Build history of the part. All positions in model axes, mm. A direction names the side the tool comes from. Round coordinates to 2 decimals unless told otherwise and drop trailing zeros. Write each loop counter-clockwise with the first axis right and the second up, starting at its lowest first coordinate (ties: lowest second). Pieces come first, ordered by that corner, then holes. Notation, with made-up numbers: (-26, -34) -> (8, -34) arc R11 cw to (8, -20) -> close; hole circle Ø3 at (-12, 38.5). An arc over 180 degrees is marked (long way). Return JSON: item names as keys, results as strings.
from build123d import *

# Parameters (mm, degrees)
SKETCH1_R           = 12
BOSS_EXTRUDE1_DEPTH = 2.94
CUT_EXTRUDE1_DEPTH  = 2.94
CUT_EXTRUDE2_DEPTH  = 2.94
SKETCH7_R           = 0.5
BOSS_EXTRUDE4_DEPTH = 9.45
SKETCH8_R           = 0.6
BOSS_EXTRUDE5_DEPTH = 0.8
SKETCH9_R           = 0.35
BOSS_EXTRUDE6_DEPTH = 0.4
SKETCH10_R          = 0.085
BOSS_EXTRUDE7_DEPTH = 0.4


with BuildPart() as part:
    # Sketch1 → Boss-Extrude1 (new body)
    with BuildSketch(Plane(origin=(0, 0, 0), x_dir=(1, 0, 0), z_dir=(0, 1, 0))):
        Circle(SKETCH1_R)
    extrude(amount=BOSS_EXTRUDE1_DEPTH)

    # Sketch2 → Cut-Extrude1 (cut)
    with BuildSketch(Plane(origin=(0, 0, 0), x_dir=(1, 0, 0), z_dir=(0, 1, 0))):
        Polygon((-11.3, 0), (-11.3, 4.756450674), (-12.628390715, 4.756450674), (-12.628390715, -4.839844075), (-11.3, -4.839844075), align=None)
        Polygon((12.628390715, -4.839844075), (12.628390715, 4.756450674), (11.3, 4.756450674), (11.3, 0), (11.3, -4.839844075), align=None)
    extrude(amount=CUT_EXTRUDE1_DEPTH, mode=Mode.SUBTRACT)

    # Sketch3 → Cut-Extrude2 (cut)
    with BuildSketch(Plane(origin=(0, 0, 0), x_dir=(1, 0, 0), z_dir=(0, 1, 0))):
        Polygon((0, -11.3), (4.998184115, -11.3), (4.998184115, -12.991968643), (-5.196787457, -12.991968643), (-5.196787457, -11.3), align=None)
        Polygon((-5.196787457, 12.991968643), (4.998184115, 12.991968643), (4.998184115, 11.3), (0, 11.3), (-5.196787457, 11.3), align=None)
    extrude(amount=CUT_EXTRUDE2_DEPTH, mode=Mode.SUBTRACT)

    # Sketch7 → Boss-Extrude4 (add)
    with BuildSketch(Plane(origin=(11.3, 0, 0), x_dir=(0, 0, -1), z_dir=(1, 0, 0))):
        with Locations((0, 1.58)):
            Circle(SKETCH7_R)
    extrude(amount=BOSS_EXTRUDE4_DEPTH)

    # Sketch8 → Boss-Extrude5 (add)
    with BuildSketch(Plane(origin=(0, 2.94, 0), x_dir=(1, 0, 0), z_dir=(0, 1, 0))):
        Circle(SKETCH8_R)
    extrude(amount=BOSS_EXTRUDE5_DEPTH)

    # Sketch9 → Boss-Extrude6 (add)
    with BuildSketch(Plane(origin=(0, 3.74, 0), x_dir=(1, 0, 0), z_dir=(0, 1, 0))):
        Circle(SKETCH9_R)
    extrude(amount=BOSS_EXTRUDE6_DEPTH)

    # Sketch10 → Boss-Extrude7 (add)
    with BuildSketch(Plane(origin=(0, 4.14, 0), x_dir=(1, 0, 0), z_dir=(0, 1, 0))):
        Circle(SKETCH10_R)
    extrude(amount=BOSS_EXTRUDE7_DEPTH)


solid = part.part
Q1. Wall check: L1, parallel to X at y = 0.6, z = -0.5; L2, parallel to Y at x = 7, z = -6; L3, parallel to Z at x = 17, y = 1.5. Give the ranges that are in metal, low to high.
Verdict:
{"L1": "x = -11.3 to 11.3", "L2": "y = 0 to 2.94", "L3": "z = -0.49 to 0.49"}
Q2. Pin check, flat tips, straight feed: pin 1 Ø2 at (x, y) = (8.5, 4) entering from +Z; pin 2 Ø4 at (x, z) = (-0.5, 3) entering from +Y; pin 3 Ø11.5 at (x, z) = (5.5, -2.5) entering from +Y; pin 4 Ø2 at (x, y) = (10, 2.5) entering from -Z. Stop position of each tip, or through.
Verdict:
{"pin 1": "passes through", "pin 2": "stops at y = 2.94", "pin 3": "stops at y = 4.14", "pin 4": "stops at z = -7.94"}
Q3. Saw through at C-C on x = 18. List the corners of the cut face in (y, z).
Verdict:
{"outline": "circle Ø1 at (1.58, 0)"}
Q4. 3-axis set-ups, long thin cutter, end or side, ignore diameter. For faces 1 (the cylindrical face through (15.959, 2.076, 0.065)), 2 (the cylindrical face through (0.323, 3.334, -0.506)), 3 (the cylindrical face through (8.54, 1.45, -8.43)): which of +Z, -Z, +X, -X, +Y, -Y reach the whole face in a straight line?
Verdict:
{"face 1": "+X", "face 2": "+Y", "face 3": "-Z, +X, +Y, -Y"}
Q5. Saw through at A-A on y = 2.4. List the corners of the cut face in (x, z), then the cut area to 3 significant figures.
Verdict:
{"outline": "(-11.3, -4.04) arc R12 ccw to (-4.04, -11.3) -> (4.04, -11.3) arc R12 ccw to (11.3, -4.04) -> (11.3, 4.04) arc R12 ccw to (4.04, 11.3) -> (-4.04, 11.3) arc R12 ccw to (-11.3, 4.04) -> close", "area": "437 mm²"}
Q6. Saw through at D-D on z = 10.25. List the corners of the cut face in (x, y), then the cut area to 3 significant figures.
Verdict:
{"outline": "(-6.24, 0) -> (6.24, 0) -> (6.24, 2.94) -> (-6.24, 2.94) -> close", "area": "36.7 mm²"}
Q7. Saw through at B-B on z = 2.25. List the corners of the cut face in (x, y).
Verdict:
{"outline": "(-11.3, 0) -> (11.3, 0) -> (11.3, 2.94) -> (-11.3, 2.94) -> close"}
